Model file for the job. Use its own axes, mm. A direction names the side the tool comes from. Round coordinates to 2 decimals unless told otherwise and drop trailing zeros. Loops run counter-clockwise (first coordinate to the right, second up) from the corner with the lowest first, then second, coordinate; pieces in that order, holes last. Notation, with made-up numbers: (38.25, 5) -> (51.25, 5) arc R13 ccw to (51.25, 17) -> close; hole circle Ø4 at (36.5, -15). An arc over 180 degrees is marked (long way). Use a Markdown table: item, result.
from build123d import *

# Parameters (mm, degrees)
BOSS_EXTRUDE1_DEPTH = 9
BEARING_HOLE_REACH  = 67.071
SKETCH11_R          = 3.175
CUT_EXTRUDE23_REACH = 67.071
SKETCH27_R          = 0.8
CUT_EXTRUDE25_DEPTH = 1.75
CUT_EXTRUDE26_REACH = 65.321
SKETCH28_R          = 2.5
CUT_EXTRUDE27_REACH = 76.071
SKETCH29_R          = 3.175
SKETCH35_W          = 33.5
SKETCH35_H          = 12.5
CUT_EXTRUDE29_DEPTH = 2
CUT_EXTRUDE30_REACH = 74.071
SKETCH36_W          = 25
SKETCH36_H          = 12.5
CUT_EXTRUDE31_REACH = 74.071
SKETCH37_R          = 1.1
FILLET1_R           = 1
SKETCH41_W          = 6
SKETCH41_H          = 12.5
BOSS_EXTRUDE4_DEPTH = 3.5
CUT_EXTRUDE32_DEPTH = 3
CUT_EXTRUDE33_DEPTH = 3
CHAMFER2_SIZE       = 0.75


with BuildPart() as part:
    # Sketch1 → Boss-Extrude1 (new body, symmetric)
    with BuildSketch(Plane(origin=(0, 0, 0), x_dir=(1, 0, 0), z_dir=(0, 1, 0))):
        Polygon((-32.535533906, 29.399494937), (-32.535533906, -29.399494937), (-24.899494937, -37.035533906), (24.899494937, -37.035533906), (32.535533906, -29.399494937), (32.535533906, 29.399494937), (24.899494937, 37.035533906), (-24.899494937, 37.035533906), align=None)
        Polygon((-25.535533906, 26.5), (-22, 30.035533906), (22, 30.035533906), (25.535533906, 26.5), (25.535533906, -26.5), (22, -30.035533906), (-22, -30.035533906), (-25.535533906, -26.5), align=None, mode=Mode.SUBTRACT)
    extrude(amount=BOSS_EXTRUDE1_DEPTH, both=True)

    # Sketch11 → Bearing Hole (cut, up to next)
    with BuildSketch(Plane(origin=(32.535533906, 0, 0), x_dir=(0, 0, -1), z_dir=(1, 0, 0)), mode=Mode.PRIVATE) as bearing_hole_sk1:
        Circle(SKETCH11_R)
    bearing_hole_tool1 = extrude(bearing_hole_sk1.sketch, amount=-BEARING_HOLE_REACH, mode=Mode.PRIVATE) & part.part
    add(bearing_hole_tool1.solids().sort_by_distance((32.535534, 0, 0))[0], mode=Mode.SUBTRACT)

    # Sketch27 → Cut-Extrude23 (cut, up to next)
    with BuildSketch(Plane.ZY.offset(32.535533906), mode=Mode.PRIVATE) as cut_extrude23_sk1:
        with Locations((-15, 0)):
            Circle(SKETCH27_R)
    cut_extrude23_tool1 = extrude(cut_extrude23_sk1.sketch, amount=-CUT_EXTRUDE23_REACH, mode=Mode.PRIVATE) & part.part
    add(cut_extrude23_tool1.solids().sort_by_distance((-32.535534, 0, -15))[0], mode=Mode.SUBTRACT)
    # Sketch27 → Cut-Extrude23 (cut, up to next)
    with BuildSketch(Plane.ZY.offset(32.535533906), mode=Mode.PRIVATE) as cut_extrude23_sk2:
        with Locations((15, 0)):
            Circle(SKETCH27_R)
    cut_extrude23_tool2 = extrude(cut_extrude23_sk2.sketch, amount=-CUT_EXTRUDE23_REACH, mode=Mode.PRIVATE) & part.part
    add(cut_extrude23_tool2.solids().sort_by_distance((-32.535534, 0, 15))[0], mode=Mode.SUBTRACT)

    # Sketch25 → Cut-Extrude25 (cut)
    with BuildSketch(Plane.ZY.offset(32.535533906)):
        with BuildLine():
            Line((-15.35, 3.48245603), (-0.5, 4.974937186))
            ThreePointArc((-0.5, 4.974937186), (0, 5), (0.5, 4.974937186))
            Line((0.5, 4.974937186), (15.35, 3.48245603))
            ThreePointArc((15.35, 3.48245603), (18.5, 0), (15.35, -3.48245603))
            Line((15.35, -3.48245603), (0.5, -4.974937186))
            ThreePointArc((0.5, -4.974937186), (0, -5), (-0.5, -4.974937186))
            Line((-0.5, -4.974937186), (-15.35, -3.48245603))
            ThreePointArc((-15.35, -3.48245603), (-18.5, 0), (-15.35, 3.48245603))
        make_face()
    extrude(amount=-CUT_EXTRUDE25_DEPTH, mode=Mode.SUBTRACT)

    # Sketch28 → Cut-Extrude26 (cut, up to next)
    with BuildSketch(Plane.ZY.offset(30.785533906), mode=Mode.PRIVATE) as cut_extrude26_sk1:
        Circle(SKETCH28_R)
    cut_extrude26_tool1 = extrude(cut_extrude26_sk1.sketch, amount=-CUT_EXTRUDE26_REACH, mode=Mode.PRIVATE) & part.part
    add(cut_extrude26_tool1.solids().sort_by_distance((-30.785534, 0, 0))[0], mode=Mode.SUBTRACT)

    # Sketch29 → Cut-Extrude27 (cut, up to next)
    with BuildSketch(Plane(origin=(0, 0, -37.035533906), x_dir=(-1, 0, 0), z_dir=(0, 0, -1)), mode=Mode.PRIVATE) as cut_extrude27_sk1:
        Circle(SKETCH29_R)
    cut_extrude27_tool1 = extrude(cut_extrude27_sk1.sketch, amount=-CUT_EXTRUDE27_REACH, mode=Mode.PRIVATE) & part.part
    add(cut_extrude27_tool1.solids().sort_by_distance((0, 0, -37.035534))[0], mode=Mode.SUBTRACT)

    # Sketch35 → Cut-Extrude29 (cut)
    with BuildSketch(Plane.XY.offset(37.035533906)):
        with Locations((5.83, 0)):
            Rectangle(SKETCH35_W, SKETCH35_H)
    extrude(amount=-CUT_EXTRUDE29_DEPTH, mode=Mode.SUBTRACT)

    # Sketch36 → Cut-Extrude30 (cut, up to next)
    with BuildSketch(Plane.XY.offset(35.035533906), mode=Mode.PRIVATE) as cut_extrude30_sk1:
        with Locations((5.83, 0)):
            Rectangle(SKETCH36_W, SKETCH36_H)
    cut_extrude30_tool1 = extrude(cut_extrude30_sk1.sketch, amount=-CUT_EXTRUDE30_REACH, mode=Mode.PRIVATE) & part.part
    add(cut_extrude30_tool1.solids().sort_by_distance((5.83, 0, 35.035534))[0], mode=Mode.SUBTRACT)

    # Sketch37 → Cut-Extrude31 (cut, up to next)
    with BuildSketch(Plane.XY.offset(35.035533906), mode=Mode.PRIVATE) as cut_extrude31_sk1:
        with Locations((19.9905, 0)):
            Circle(SKETCH37_R)
    cut_extrude31_tool1 = extrude(cut_extrude31_sk1.sketch, amount=-CUT_EXTRUDE31_REACH, mode=Mode.PRIVATE) & part.part
    add(cut_extrude31_tool1.solids().sort_by_distance((19.9905, 0, 35.035534))[0], mode=Mode.SUBTRACT)
    # Sketch37 → Cut-Extrude31 (cut, up to next)
    with BuildSketch(Plane.XY.offset(35.035533906), mode=Mode.PRIVATE) as cut_extrude31_sk2:
        with Locations((-8.3305, 0)):
            Circle(SKETCH37_R)
    cut_extrude31_tool2 = extrude(cut_extrude31_sk2.sketch, amount=-CUT_EXTRUDE31_REACH, mode=Mode.PRIVATE) & part.part
    add(cut_extrude31_tool2.solids().sort_by_distance((-8.3305, 0, 35.035534))[0], mode=Mode.SUBTRACT)

    # Fillet1
    fillet1_edges = [part.edges().sort_by_distance(p)[0] for p in [
        (22.58, 6.25, 36.035533906),
        (22.58, -6.25, 36.035533906),
        (-10.92, -6.25, 36.035533906),
        (-10.92, 6.25, 36.035533906),
        (18.33, 6.25, 32.535533906),
        (18.33, -6.25, 32.535533906),
        (-6.67, 6.25, 32.535533906),
    ]]
    fillet(fillet1_edges, radius=FILLET1_R)

    # Sketch41 → Boss-Extrude4 (add)
    with BuildSketch(Plane(origin=(0, 0, 30.035533906), x_dir=(-1, 0, 0), z_dir=(0, 0, -1))):
        with Locations((-15.33, 0)):
            Rectangle(SKETCH41_W, SKETCH41_H)
    extrude(amount=-BOSS_EXTRUDE4_DEPTH)

    # Sketch42 → Cut-Extrude32 (cut)
    with BuildSketch(Plane(origin=(-25.535533906, 0, 0), x_dir=(0, 0, -1), z_dir=(1, 0, 0))):
        Polygon((-12.75, -1.299038106), (-12.75, 1.299038106), (-15, 2.598076211), (-17.25, 1.299038106), (-17.25, -1.299038106), (-15, -2.598076211), align=None)
        Polygon((17.25, 1.299038106), (15, 2.598076211), (12.75, 1.299038106), (12.75, -1.299038106), (15, -2.598076211), (17.25, -1.299038106), align=None)
    extrude(amount=-CUT_EXTRUDE32_DEPTH, mode=Mode.SUBTRACT)

    # Sketch43 → Cut-Extrude33 (cut)
    with BuildSketch(Plane(origin=(0, 0, 30.035533906), x_dir=(-1, 0, 0), z_dir=(0, 0, -1))):
        Polygon((-17.7405, -1.299038106), (-17.7405, 1.299038106), (-19.9905, 2.598076211), (-22.2405, 1.299038106), (-22.2405, -1.299038106), (-19.9905, -2.598076211), align=None)
        Polygon((6.0805, -1.299038106), (8.3305, -2.598076211), (10.5805, -1.299038106), (10.5805, 1.299038106), (8.3305, 2.598076211), (6.0805, 1.299038106), align=None)
    extrude(amount=-CUT_EXTRUDE33_DEPTH, mode=Mode.SUBTRACT)

    # Chamfer2
    chamfer2_edges = [part.edges().sort_by_distance(p)[0] for p in [
        (-28.717514421, 9, 33.217514421),
        (-32.535533906, -9, 0),
        (-28.717514421, -9, -33.217514421),
        (28.717514421, 9, 33.217514421),
        (32.535533906, 9, 0),
        (28.717514421, 9, -33.217514421),
        (0, 9, -37.035533906),
        (-25.535533906, -9, 0),
        (-23.767766953, -9, 28.267766953),
        (23.767766953, -9, 28.267766953),
        (25.535533906, -9, 0),
        (23.767766953, -9, -28.267766953),
        (0, -9, -30.035533906),
        (-23.767766953, -9, -28.267766953),
        (-25.535533906, 9, 0),
        (-23.767766953, 9, 28.267766953),
        (23.767766953, 9, 28.267766953),
        (25.535533906, 9, 0),
        (23.767766953, 9, -28.267766953),
        (0, 9, -30.035533906),
        (-23.767766953, 9, -28.267766953),
        (-28.717514421, 9, -33.217514421),
        (-32.535533906, 9, 0),
        (0, -9, -37.035533906),
        (28.717514421, -9, -33.217514421),
        (32.535533906, -9, 0),
        (28.717514421, -9, 33.217514421),
        (-28.717514421, -9, 33.217514421),
    ]]
    chamfer(chamfer2_edges, length=CHAMFER2_SIZE)


solid = part.part
Q1. Band-saw the part on C-C, the plane x = 11.5. Give the cut face in (y, z), plus the area to 3 significant figures.
Results list:
| item | result |
|---|---|
| outline | (-9, -36.29) -> (-8.25, -37.04) -> (8.25, -37.04) -> (9, -36.29) -> (9, -30.79) -> (8.25, -30.04) -> (-8.25, -30.04) -> (-9, -30.79) -> close; (-9, 30.04) -> (-6.25, 30.04) -> (-6.25, 37.04) -> (-9, 37.04) -> close; (6.25, 30.04) -> (9, 30.04) -> (9, 37.04) -> (6.25, 37.04) -> close |
| area | 163 mm² |
Q2. Flat gauge pins, fed straight in: pin 1 (3 mm diameter, centred on x = -26.5, y = -0.5, fed in from +Z) (3 decimals); pin 2 (0.8 mm diameter, centred on y = -2.5, z = 34, fed in from -X) (3 decimals); pin 3 (1 mm diameter, centred on y = 2, z = 32, fed in from -X) (3 decimals); pin 4 (3 mm diameter, centred on x = 24, z = -9.5, fed in from +Y). Where does each tip first touch, or does it go through?
Results list:
| item | result |
|---|---|
| pin 1 | stops at z = 36.935 |
| pin 2 | stops at x = -28.335 |
| pin 3 | stops at x = -30.435 |
| pin 4 | passes through |
Q3. Band-saw the part on A-A, the plane x = 0. Give the cut face in (y, z) (3 decimals).
Results list:
| item | result |
|---|---|
| outline | (-9, -36.286) -> (-8.25, -37.036) -> (-3.175, -37.036) -> (-3.175, -30.036) -> (-8.25, -30.036) -> (-9, -30.786) -> close; (-9, 30.036) -> (-6.25, 30.036) -> (-6.25, 37.036) -> (-9, 37.036) -> close; (3.175, -37.036) -> (8.25, -37.036) -> (9, -36.286) -> (9, -30.786) -> (8.25, -30.036) -> (3.175, -30.036) -> close; (6.25, 30.036) -> (9, 30.036) -> (9, 37.036) -> (6.25, 37.036) -> close |
Q4. Drill centre lines: L1, parallel to Z at x = 2.5, y = 8.25; L2, parallel to X at y = -1, z = 20; L3, parallel to Y at x = 30.75, z = 0 (3 decimals). Where is each one in solid material? Low to high. Write a range as from..to.
Results list:
| item | result |
|---|---|
| L1 | z = -37.04..-30.04, 30.04..37.04 |
| L2 | x = -32.54..-25.54, 25.54..32.54 |
| L3 | y = -9..-3.175, 3.175..9 |
Q5. Tool access for faces 4 (the face through (-30.786, -3, 0)), 5 (the face through (22, 0, 35.036)), 6 (the face through (21.13, -1.94, 31.51)), 7 (the face through (-23.793, 0.116, -28.243)): list every direction of +Z, -Z, +X, -X, +Y, -Y with a clear straight run to the whole face (end or side of a thin tool).
Results list:
| item | result |
|---|---|
| face 4 | -X |
| face 5 | +Z |
| face 6 | none |
| face 7 | +Y, -Y |
Q6. Band-saw the part on D-D, the plane z = 9.5. Give the cut face in (x, y).
Results list:
| item | result |
|---|---|
| outline | (-32.54, -8.25) -> (-31.79, -9) -> (-26.29, -9) -> (-25.54, -8.25) -> (-25.54, 8.25) -> (-26.29, 9) -> (-31.79, 9) -> (-32.54, 8.25) -> (-32.54, 4.07) -> (-30.79, 4.07) -> (-30.79, -4.07) -> (-32.54, -4.07) -> close; (25.54, -8.25) -> (26.29, -9) -> (31.79, -9) -> (32.54, -8.25) -> (32.54, 8.25) -> (31.79, 9) -> (26.29, 9) -> (25.54, 8.25) -> close |
Q7. Band-saw the part on B-B, the plane z = -24. Give the cut face in (x, y).
Results list:
| item | result |
|---|---|
| outline | (-32.54, -8.25) -> (-31.79, -9) -> (-26.29, -9) -> (-25.54, -8.25) -> (-25.54, 8.25) -> (-26.29, 9) -> (-31.79, 9) -> (-32.54, 8.25) -> close; (25.54, -8.25) -> (26.29, -9) -> (31.79, -9) -> (32.54, -8.25) -> (32.54, 8.25) -> (31.79, 9) -> (26.29, 9) -> (25.54, 8.25) -> close |
Q8. Pull direction Z, two halves, no side cores. Call faces 1 (the face through (-28.4, 8.62, -33.01)), 2 (the face through (-27, 0, 17.25)), 3 (the face through (-32.536, 6, 0)): released by +Z, released by -Z, zero draft, split by the parting line, or undercut.
Results list:
| item | result |
|---|---|
| face 1 | released by -Z |
| face 2 | undercut |
| face 3 | zero draft |
